Work out the finished part from the listing and answer in its coordinate system (mm). Face numbers are marked on the shaded views. Give positions to 0.01 mm unless a question says otherwise; leave off trailing zeros. Order: outer loops, then holes, each group sorted by start corner. A loop starts at its lowest first (then second) coordinate and runs counter-clockwise, first axis right, second up. Notation, with made-up numbers: (76, 14.5) -> (87, 14.5) arc R25 ccw to (87, 40.5) -> close; hole circle Ø4 at (-38.5, 30). An arc over 180 degrees is marked (long way). Use a Markdown table: item, result. Add a question column.
```python
from build123d import *

# Parameters (mm, degrees)
F0_R     = 35.391542
F1_DEPTH = 5
F3_R     = 1.682004
F4_DEPTH = 25
F5_R     = 1.935057
F6_DEPTH = 25
F7_R     = 1.754642
F8_DEPTH = 25
F2_W     = 4.903845
F2_H     = 30.000002
F9_DEPTH = 3


with BuildPart() as f1:
    # F0 (on Front) → F1 (new body)
    with BuildSketch(Plane.XZ):
        Circle(F0_R)
    extrude(amount=F1_DEPTH)

    # F3 (on face) → F4 (cut)
    with BuildSketch(Plane.XZ.offset(5)):
        with Locations((0, -10.961539)):
            Circle(F3_R)
    extrude(amount=-F4_DEPTH, mode=Mode.SUBTRACT)

    # F5 (on face) → F6 (cut)
    with BuildSketch(Plane.XZ.offset(5)):
        with Locations((0, 11.250001)):
            Circle(F5_R)
    extrude(amount=-F6_DEPTH, mode=Mode.SUBTRACT)

    # F7 (on face) → F8 (cut)
    with BuildSketch(Plane.XZ.offset(5)):
        Circle(F7_R)
    extrude(amount=-F8_DEPTH, mode=Mode.SUBTRACT)

    # F2 (on face) → F9 (join)
    with BuildSketch(Plane.XZ.offset(5)):
        with Locations((-18.317308, 0)):
            Rectangle(F2_W, F2_H)
    extrude(amount=F9_DEPTH)


solid = f1.part
```
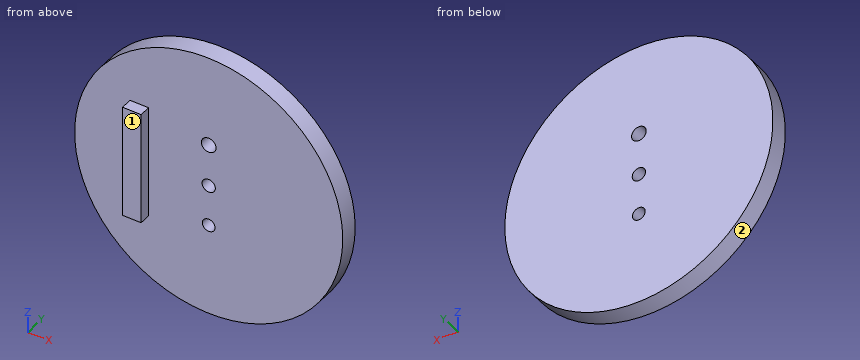
1) The part is cut by section A-A, the plane z = 0. Determine the outline of the cut face in (x, y), then the cut area to 3 significant figures.
2) The part is cut by section D-D, the plane y = -2.5. Determine the outline of the cut face in (x, z), then the cut area to 3 significant figures.
3) Flat-ended cylindrical pins translate along their axes: pin 1 (3 mm diameter, centred on y = -6, z = -22, fed in from +X); pin 2 (1.5 mm diameter, centred on x = -17.5, y = -6.5, fed in from +Z); pin 3 (2 mm diameter, centred on y = -3, z = -6.5, fed in from +X). Find the tip coordinate at first contact, or state that the pin passes through.
4) The part is cut by section B-B, the plane x = 0. Determine the outline of the cut face in (y, z).
5) Determine the mould class of the marked faces 1 and 2 for opening direction Z: released by +Z, released by -Z, zero draft, split by the parting line, or undercut.
6) The part is cut by section C-C, the plane z = -14. Determine the outline of the cut face in (x, y), then the cut area to 3 significant figures.
7) Straight lines are drawn through the part: line 1 (Z direction, x = 0, y = -2.45); line 2 (X direction, y = -7.25, z = 4); line 3 (Y direction, x = 3, z = 1). For each, find the intervals that lie inside material, in ascending order.
A:
| question | item | result |
|---|---|---|
| 1 | outline | (-35.39, -5) -> (-20.77, -5) -> (-20.77, -8) -> (-15.87, -8) -> (-15.87, -5) -> (-1.75, -5) -> (-1.75, 0) -> (-35.39, 0) -> close; (1.75, -5) -> (35.39, -5) -> (35.39, 0) -> (1.75, 0) -> close |
| 1 | area | 351 mm^2 |
| 2 | outline | circle Ø70.78 at (0, 0); hole circle Ø3.87 at (0, 11.25); hole circle Ø3.51 at (0, 0); hole circle Ø3.36 at (0, -10.96) |
| 2 | area | 3,900 mm^2 |
| 3 | pin 1 | x = 28.57 |
| 3 | pin 2 | z = 15 |
| 3 | pin 3 | x = 34.96 |
| 4 | outline | (-5, -35.39) -> (0, -35.39) -> (0, -12.64) -> (-5, -12.64) -> close; (-5, -9.28) -> (0, -9.28) -> (0, -1.75) -> (-5, -1.75) -> close; (-5, 1.75) -> (0, 1.75) -> (0, 9.31) -> (-5, 9.31) -> close; (-5, 13.19) -> (0, 13.19) -> (0, 35.39) -> (-5, 35.39) -> close |
| 5 | face 1 | zero draft |
| 5 | face 2 | split by the parting line |
| 6 | outline | (-32.5, -5) -> (-20.77, -5) -> (-20.77, -8) -> (-15.87, -8) -> (-15.87, -5) -> (32.5, -5) -> (32.5, 0) -> (-32.5, 0) -> close |
| 6 | area | 340 mm^2 |
| 7 | line 1 | -35.39 to -12.64, -9.28 to -1.75, 1.75 to 9.31, 13.19 to 35.39 |
| 7 | line 2 | -20.77 to -15.87 |
| 7 | line 3 | -5 to 0 |
